Design review of the part built by this model. Coordinates are the model's own, in mm. Face numbers are marked on the shaded views. A direction names the side the tool comes from. Coordinates: 2 decimals unless noted, no trailing zeros. Order: outer loops, then holes, each group sorted by start corner. A loop starts at its lowest first (then second) coordinate and runs counter-clockwise, first axis right, second up. Notation, with made-up numbers: M 61.5,85.5 L 73.5,85.5 A18 ccw 73.5,118.5 Z; hole C -38.75,-32 d1. An arc over 180 degrees is marked long. Use CSV: the item, a comma, the result in double quotes.
```python
from build123d import *

# Parameters (mm, degrees)
PAD_DEPTH       = 5
SKETCH001_W     = 80
SKETCH001_H     = 14.2
POCKET_DEPTH    = 1.5
SKETCH002_R     = 2.3
POCKET001_DEPTH = 3


with BuildPart() as part:
    # Sketch → Pad (new body)
    with BuildSketch(Plane.XY):
        with BuildLine():
            ThreePointArc((8, 16), (0, 8), (8, 0))
            Line((42, 0), (8, 0))
            ThreePointArc((42, 0), (50, 8), (42, 16))
            Line((8, 16), (42, 16))
        make_face()
    extrude(amount=PAD_DEPTH)

    # Sketch001 (on Face6 of Pad) → Pocket (cut)
    with BuildSketch(Plane.XY.offset(5)):
        with Locations((40, 8.1)):
            Rectangle(SKETCH001_W, SKETCH001_H)
    extrude(amount=-POCKET_DEPTH, mode=Mode.SUBTRACT)

    # Sketch002 (on Face2 of Pocket) → Pocket001 (cut)
    with BuildSketch(Plane(origin=(0, 0, 0), x_dir=(1, 0, 0), z_dir=(0, 0, -1))):
        with Locations((8, -8)):
            Circle(SKETCH002_R)
    extrude(amount=-POCKET001_DEPTH, mode=Mode.SUBTRACT)


solid = part.part
```
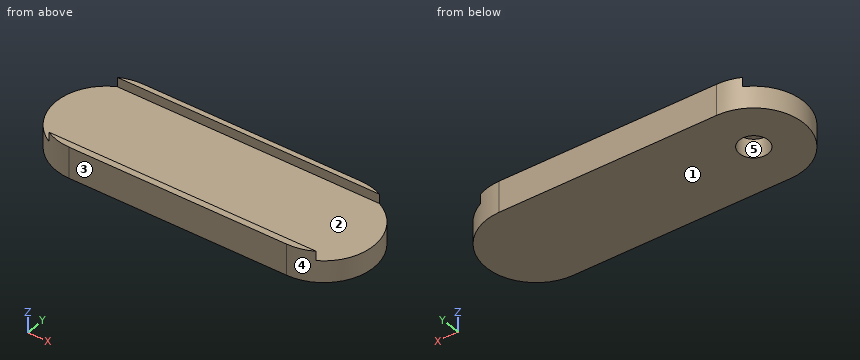
(1) Add section C-C on x = 19. State the section outline as (y, z) points, and give its area (3 significant figures).
The answers:
outline,"M 0,0 L 16,0 L 16,5 L 15.2,5 L 15.2,3.5 L 1,3.5 L 1,5 L 0,5 Z"
area,"58.7 mm2"
(2) Wall thickness on probe 1 along Y at (x, z) = (8, 1.9); probe 2 along Y at (x, z) = (20, 3.95); probe 3 along X at (y, z) = (8, 1.5): over which ranges is each line inside the solid? List them lowest first.
The answers:
probe 1,"y = 0 to 5.7, 10.3 to 16"
probe 2,"y = 0 to 1, 15.2 to 16"
probe 3,"x = 0 to 5.7, 10.3 to 50"
(3) The part is to be moulded in two halves that separate along Y. For the marked faces 1, 2 and 3, say which applies: pulls with the +Y half, pulls with the -Y half, needs draft (parallel to the pull), parting line crosses it, or undercut.
The answers:
face 1,"needs draft"
face 2,"undercut"
face 3,"pulls with the -Y half"
(4) Add section A-A on z = 4.3. State the section outline as (x, y) points.
The answers:
outline,"M 4.13,1 A8 ccw 8,0 L 42,0 A8 ccw 45.87,1 Z; M 4.51,15.2 L 45.49,15.2 A8 ccw 42,16 L 8,16 A8 ccw Z"
(5) Clearance check with flat-ended pins moving along their axes: P1, Ø1, axis at y = 2.5, z = 2.5, coming from the +X side (3 decimals); P2, Ø6, axis at x = 44.5, y = 6, coming from the +Z side; P3, Ø1.5, axis at y = 12.5, z = 2.5, coming from the -X side. State where each tip first meets the part, or that it passes through.
The answers:
P1,"stops at x = 48.245"
P2,"stops at z = 3.5"
P3,"stops at x = 0.93"
(6) For the marked faces 4 and 5, list the 3-axis set-ups (+Z, -Z, +X, -X, +Y, -Y) from which the entire face can be reached by the end or side of a thin tool; tool diameter is ignored.
The answers:
face 4,"+Z, -Z, +X"
face 5,"-Z"
(7) Add section B-B on y = 8. State the section outline as (x, z) points.
The answers:
outline,"M 0,0 L 5.7,0 L 5.7,3 L 10.3,3 L 10.3,0 L 50,0 L 50,3.5 L 0,3.5 Z"
(8) Add section D-D on z = 1.2. State the section outline as (x, y) points.
The answers:
outline,"M 8,0 L 42,0 A8 ccw 42,16 L 8,16 A8 ccw Z; hole C 8,8 d4.6"
